Autodesk Inventor part; units mm, degrees
ref_plane "YZ Plane" through (0, 0, 0) normal (1, 0, 0) x (0, 1, 0)
ref_plane "XZ Plane" through (0, 0, 0) normal (0, 1, 0) x (-1, 0, 0)
ref_plane "XY Plane" through (0, 0, 0) normal (0, 0, 1) x (1, 0, 0)
sketch "スケッチ1" plane through (0, 0, 0) normal (0, 0, 1) x (1, 0, 0)
  circle A0 centre (-5.2771, -42.7168) radius 0.85
  circle A1 centre (-21.2771, -42.7168) radius 0.85
  circle A2 centre (-5.2771, -6.7168) radius 0.85
  circle A3 centre (-13.2771, -13.2168) radius 8
  line L0 (-3.2771, -4.7168) -> (-7.2771, -4.7168)
  line L1 (-7.2771, -4.7168) -> (-7.2771, -44.7168)
  line L2 (-7.2771, -44.7168) -> (-3.2771, -44.7168)
  line L3 (-3.2771, -44.7168) -> (-3.2771, -4.7168)
  line L4 (-3.2771, -44.7168) -> (-23.2771, -44.7168)
  line L5 (-23.2771, -44.7168) -> (-23.2771, -40.7168)
  line L6 (-23.2771, -40.7168) -> (-3.2771, -40.7168)
  line L7 (-3.2771, -40.7168) -> (-3.2771, -44.7168)
  circle A4 centre (-5.2771, -6.7168) radius 2
  circle A5 centre (-21.2771, -42.7168) radius 2
  circle A6 centre (-5.2771, -6.7168) radius 1.1
  circle A7 centre (-5.2771, -42.7168) radius 1.1
  circle A8 centre (-21.2771, -42.7168) radius 1.1
  line L8 (-5.2771, -66.2168) -> (-21.2771, -66.2168) construction
  circle A9 centre (-5.2771, -89.7168) radius 0.85
  circle A10 centre (-21.2771, -89.7168) radius 0.85
  circle A11 centre (-5.2771, -125.7168) radius 0.85
  circle A12 centre (-13.2771, -119.2168) radius 8
  line L9 (-3.2771, -127.7168) -> (-7.2771, -127.7168)
  line L10 (-7.2771, -127.7168) -> (-7.2771, -87.7168)
  line L11 (-7.2771, -87.7168) -> (-3.2771, -87.7168)
  line L12 (-3.2771, -87.7168) -> (-3.2771, -127.7168)
  line L13 (-3.2771, -87.7168) -> (-23.2771, -87.7168)
  line L14 (-23.2771, -87.7168) -> (-23.2771, -91.7168)
  line L15 (-23.2771, -91.7168) -> (-3.2771, -91.7168)
  line L16 (-3.2771, -91.7168) -> (-3.2771, -87.7168)
  circle A13 centre (-5.2771, -125.7168) radius 2
  circle A14 centre (-21.2771, -89.7168) radius 2
  circle A15 centre (-5.2771, -125.7168) radius 1.1
  circle A16 centre (-5.2771, -89.7168) radius 1.1
  circle A17 centre (-21.2771, -89.7168) radius 1.1
  line L17 (-3.2771, -44.7168) -> (-3.2771, -87.7168)
  line L18 (-23.2771, -44.7168) -> (-23.2771, -87.7168)
  line L19 (-6.4151, -24.526) -> (-6.4151, -30.526)
  line L20 (-6.2865, -24.2474) -> (-6.2865, -30.6046)
  line L21 (-6.2865, -30.6046) -> (-10.1437, -30.6046)
  line L22 (-10.1437, -24.2474) -> (-6.2865, -24.2474)
  line L23 (-6.4151, -107.9075) -> (-6.4151, -101.9075)
  line L24 (-6.2865, -108.1861) -> (-6.2865, -101.8289)
  line L25 (-6.2865, -101.8289) -> (-10.1437, -101.8289)
  line L26 (-10.1437, -108.1861) -> (-6.2865, -108.1861)
  line L27 (7.0429, 25.428) -> (7.0429, 23.728)
  point P0 (0, 0)
  point P1 (-3.2771, -42.7168)
  point P2 (-5.2771, -4.7168)
  point P3 (-13.2771, -44.7168)
  point P4 (-13.2771, -66.2168)
  point P5 (-3.2771, -89.7168)
  point P6 (-5.2771, -127.7168)
  point P7 (-13.2771, -87.7168)
  point P8 (-7.2771, -6.7168)
  point P9 (-7.2771, -7.9253)
  point P10 (-7.2771, -18.5083)
  point P11 (-7.2771, -40.7168)
  point P12 (-21.2771, -40.7168)
  point P13 (-23.2771, -42.7168)
  point P14 (-23.2771, -89.7168)
  point P15 (-21.2771, -91.7168)
  point P16 (-7.2771, -91.7168)
  point P17 (-7.2771, -113.9253)
  point P18 (-7.2771, -124.5083)
  point P19 (-7.2771, -125.7168)
  point P20 (-3.2771, -125.7168)
  point P21 (-3.2771, -6.7168)
  point P22 (-7.2771, -24.2474)
  point P23 (-7.2771, -30.6046)
  point P24 (-7.2771, -101.8289)
  point P25 (-7.2771, -108.1861)
  point P26 (7.0429, 24.578)
  dimension "d0" = 4
  dimension "d1" = 4
  dimension "d2" = 2.2
  dimension "d3" = 2.2
  dimension "d4" = 2.2
  dimension "d11" = 53
extrude "押し出し1" add sketch "スケッチ1" along normal blind 1.5 contours A3 L1 A4 L3 L6 L21 L20 L22 | A4 | L3 L2 L1 L6 | L1 L4 A5 L6 | L17 L11 L13 L18 L4 L2 | A5 | L12 L15 L10 L11 | L4 L5 A5 | L10 L15 A14 L13 | L12 A13 L10 A12 L26 L24 L25 L15 | A14 L14 L13 | A14 | A13
fillet "フィレット1" radius 2 4 edges at (-7.2771, -108.1861, 0.75) (-7.2771, -101.8289, 0.75) (-7.2771, -24.2474, 0.75) (-7.2771, -30.6046, 0.75)
fillet "フィレット2" radius 2 4 edges at (-7.2771, -18.5083, 0.75) (-7.2771, -7.9253, 0.75) (-7.2771, -124.5083, 0.75) (-7.2771, -113.9253, 0.75)
fillet "フィレット3" radius 3 2 edges at (-7.2771, -91.7168, 0.75) (-7.2771, -40.7168, 0.75)
sketch "スケッチ2" plane through (0, 0, 1.5) normal (0, 0, 1) x (1, 0, 0)
  circle A0 centre (-6.2771, -47.7168) radius 1.1
  line L0 (-3.2771, -125.7168) -> (-3.2771, -6.7168)
  circle A1 centre (-5.2771, -42.7168) radius 1.1
  circle A2 centre (-20.2771, -47.7168) radius 1.1
  line L1 (-23.2771, -42.7168) -> (-23.2771, -89.7168)
  line L2 (-3.2771, -66.2168) -> (-23.2771, -66.2168) construction
  circle A3 centre (-6.2771, -84.7168) radius 1.1
  circle A4 centre (-20.2771, -84.7168) radius 1.1
  line L3 (-20.2771, -52.7168) -> (-6.2771, -52.7168)
  line L4 (-6.2771, -52.7168) -> (-6.2771, -79.7168)
  line L5 (-6.2771, -79.7168) -> (-20.2771, -79.7168)
  line L6 (-20.2771, -79.7168) -> (-20.2771, -52.7168)
  line L7 (-20.2771, -52.7168) -> (-6.2771, -79.7168) construction
  line L8 (-6.2771, -52.7168) -> (-20.2771, -79.7168) construction
  point P0 (0, 0)
  point P1 (-13.2771, -66.2168)
  dimension "d12" = 2.2
  dimension "d13" = 3
  dimension "d14" = 5
  dimension "d15" = 2.2
  dimension "d16" = 3
  dimension "d17" = 5
  dimension "d18" = 3
extrude "押し出し2" cut sketch "スケッチ2" against normal blind 1.5 contours A0 | A2 | A3 | A4 | L3 L4 L5 L6
fillet "フィレット4" radius 3 4 edges at (-20.2771, -52.7168, 0.75) (-6.2771, -52.7168, 0.75) (-20.2771, -79.7168, 0.75) (-6.2771, -79.7168, 0.75)
equation "\"d16\" = d13"
properties part number "new_ude" material "アルミニウム 2014-T4"
The listing builds one solid part. Answer for the finished solid, in the listing's coordinates (mm). A direction names the side the tool comes from. Coordinates: 2 decimals unless noted, no trailing zeros. Write each loop counter-clockwise with the first axis right and the second up, starting at its lowest first coordinate (ties: lowest second). Pieces come first, ordered by that corner, then holes. Notation, with made-up numbers: M 59,9.25 L 99,9.25 A29 cw 99,33.25 Z; hole C 9.5,70 d3. An arc over 180 degrees is marked long. Use a Markdown table: item, result. Add a question column.
1. Section D-D (y = -118) is taken. Give the vertices of the cut face in (x, z), plus the area to 3 significant figures.
2. Section C-C (z = 0.95) is taken. Count the separate pieces of the cut face and the enclosed holes in it, plus the area to 3 significant figures.
3. Which of the six approach directions +Z, -Z, +X, -X, +Y, -Y give full straight-line access (tool end or side, diameter ignored) to faces 1 (the cylindrical face through (-19.42, -53.62, 0.74)), 2 (the cylindrical face through (-5.321, -4.717, 0.74))?
4. Given P1, Ø0.8, axis at y = -21.5, z = 0.5, coming from the -X side, flat-ended and moving along its own axis, determine where the tip first touches the part or whether it passes through.
5. Straight lines are drawn through the part: line 1 along Y through (x, z) = (-13, 1.45); line 2 along Y through (x, z) = (-20.5, 0.3); line 3 along X through (y, z) = (-43, 0.1). For each, find the intervals that lie inside material, in ascending order. Write a range as [from, to].
6. For a pull along Y with two mould halves and no side action, classify faces 3 (the flat face through (-4, -66, 0)), 4 (the cylindrical face through (-22.676, -91.146, 0.74)), 5 (the cylindrical face through (-7.18, -53.57, 0.74)) as +Y half, -Y half, draft (parallel to the pull), parting line (faces both ways), or undercut.
7. Section B-B (x = -12) is taken. Give the vertices of the cut face in (y, z), plus the area to 3 significant figures.
8. Section A-A (y = -62) is taken. Give the vertices of the cut face in (x, z).
Data:
| question | item | result |
|---|---|---|
| 1 | outline | M -5.37,0 L -3.28,0 L -3.28,1.5 L -5.37,1.5 Z |
| 1 | area | 3.14 mm2 |
| 2 | separate pieces | 1 |
| 2 | enclosed holes | 11 |
| 2 | area | 855 mm2 |
| 3 | face 1 | +Z, -Z |
| 3 | face 2 | +Z, -Z, +Y |
| 4 | P1 | stops at x = -7.28 |
| 5 | line 1 | y = [-91.72, -79.72], [-52.72, -40.72] |
| 5 | line 2 | y = [-91.72, -90.5], [-88.94, -85.79], [-83.64, -48.79], [-46.64, -43.5], [-41.94, -40.72] |
| 5 | line 3 | x = [-23.28, -22.34], [-20.21, -6.34], [-4.21, -3.28] |
| 6 | face 3 | draft |
| 6 | face 4 | -Y half |
| 6 | face 5 | undercut |
| 7 | outline | M -91.72,0 L -79.72,0 L -79.72,1.5 L -91.72,1.5 Z; M -52.72,0 L -40.72,0 L -40.72,1.5 L -52.72,1.5 Z |
| 7 | area | 36.0 mm2 |
| 8 | outline | M -23.28,0 L -20.28,0 L -20.28,1.5 L -23.28,1.5 Z; M -6.28,0 L -3.28,0 L -3.28,1.5 L -6.28,1.5 Z |
